Check sheet for the modelled part. Datum: model origin and axes. Units: mm. Coordinates: 2 decimals unless noted, no trailing zeros. Loops run counter-clockwise (first coordinate to the right, second up) from the corner with the lowest first, then second, coordinate; pieces in that order, holes last. Notation, with made-up numbers: (-0.5, 42.5) -> (28.5, 42.5) arc R10 ccw to (28.5, 59.5) -> close; hole circle Ø10 at (21, 28.5). An arc over 180 degrees is marked (long way). Use one line per item in the form item = value.
Autodesk Inventor part; units mm, degrees
ref_plane "YZ Plane" through (0, 0, 0) normal (1, 0, 0) x (0, 1, 0)
ref_plane "XZ Plane" through (0, 0, 0) normal (0, 1, 0) x (-1, 0, 0)
ref_plane "XY Plane" through (0, 0, 0) normal (0, 0, 1) x (1, 0, 0)
sketch "スケッチ1" plane through (0, 0, 0) normal (0, 1, 0) x (-1, 0, 0)
  circle A0 centre (0, 0) radius 5.05
  line L0 (-8.5, 0) -> (8.5, 0) construction
  circle A1 centre (-8.5, 0) radius 1.35
  circle A2 centre (-6.0104, -6.0104) radius 1.35
  circle A3 centre (0, -8.5) radius 1.35
  circle A4 centre (6.0104, -6.0104) radius 1.35
  circle A5 centre (0, -145.8097) radius 16 construction
  line L1 (0, 0) -> (0, -145.8097) construction
  arc A6 (-20.3699, -115.9088) -> (20.3699, -115.9088) centre (0, -145.8097) ccw
  circle A7 centre (-8.5, 0) radius 2.4 construction
  line L2 (-16, 31) -> (16, 31) construction
  line L3 (16, 31) -> (16, -12) construction
  line L4 (16, -12) -> (-16, -12) construction
  line L5 (-16, -12) -> (-16, 31) construction
  line L6 (-16, 31) -> (16, -12) construction
  line L7 (16, 31) -> (-16, -12) construction
  arc A8 (-16, 0) -> (-10.583, -12) centre (0, 0) ccw construction
  arc A9 (10.583, -12) -> (16, 0) centre (0, 0) ccw construction
  line L8 (-16, -107.6443) -> (-16, 0)
  line L9 (16, -107.6443) -> (16, 0)
  circle A10 centre (0, -82.5) radius 1.6
  line L10 (0, -145.8097) -> (-25.5832, -120.2265) construction
  circle A11 centre (-22.7548, -123.055) radius 4 construction
  circle A12 centre (-22.7548, -123.055) radius 1.6
  circle A13 centre (-22.7548, -168.5645) radius 1.6
  circle A14 centre (22.7548, -168.5645) radius 1.6
  circle A15 centre (22.7548, -123.055) radius 1.6
  line L11 (30.6064, -21.0119) -> (2.8936, -37.0119) construction
  line L12 (2.8936, -37.0119) -> (-18.6064, 0.2272) construction
  line L13 (-18.6064, 0.2272) -> (9.1064, 16.2272) construction
  line L14 (9.1064, 16.2272) -> (30.6064, -21.0119) construction
  line L15 (30.6064, -21.0119) -> (-18.6064, 0.2272) construction
  line L16 (2.8936, -37.0119) -> (9.1064, 16.2272) construction
  line L17 (16.75, -29.0119) -> (-4.75, 8.2272) construction
  circle A16 centre (0, -42.5) radius 1.6
  line L18 (-2.5, -47.5) -> (2.5, -47.5) construction
  line L19 (2.5, -47.5) -> (2.5, -57.5) construction
  line L20 (2.5, -57.5) -> (-2.5, -57.5) construction
  line L21 (-2.5, -57.5) -> (-2.5, -47.5) construction
  line L22 (-2.5, -47.5) -> (2.5, -57.5) construction
  line L23 (2.5, -47.5) -> (-2.5, -57.5) construction
  line L24 (-2.5, -52.5) -> (2.5, -52.5) construction
  circle A17 centre (0, -62.5) radius 1.6
  line L25 (2.8936, -37.0119) -> (49.2811, -117.3573) construction
  line L26 (0, -145.8097) -> (49.2811, -117.3573) construction
  line L27 (-2.5, -47.5) -> (2.5, -47.5) construction
  line L28 (2.5, -47.5) -> (2.5, -77.5) construction
  line L29 (2.5, -77.5) -> (-2.5, -77.5) construction
  line L30 (-2.5, -77.5) -> (-2.5, -47.5) construction
  line L31 (-2.5, -47.5) -> (2.5, -77.5) construction
  line L32 (2.5, -47.5) -> (-2.5, -77.5) construction
  line L33 (-2.55, -47.45) -> (2.55, -47.45)
  line L34 (2.55, -47.45) -> (2.55, -77.55)
  line L35 (2.55, -77.55) -> (-2.55, -77.55)
  line L36 (-2.55, -77.55) -> (-2.55, -47.45)
  line L37 (-2.55, -47.45) -> (2.55, -77.55) construction
  line L38 (2.55, -47.45) -> (-2.55, -77.55) construction
  arc A18 (-1.0651, -47.45) -> (-2.55, -48.9349) centre (-1.8075, -48.1925) ccw
  arc A19 (2.55, -48.9349) -> (1.0651, -47.45) centre (1.8075, -48.1925) ccw
  line L39 (-2.5, -62.5) -> (2.5, -62.5) construction
  arc A20 (-2.55, -76.0651) -> (-1.0651, -77.55) centre (-1.8075, -76.8075) ccw
  arc A21 (1.0651, -77.55) -> (2.55, -76.0651) centre (1.8075, -76.8075) ccw
  arc A22 (16, 0) -> (8.0571, 13.8233) centre (0, 0) ccw
  circle A23 centre (0, -145.8097) radius 28.1801
  line L40 (-5.05, 0) -> (-5.05, 12.0954)
  line L41 (5.05, 0) -> (5.05, 12.0954)
  circle A24 centre (8.5, 0) radius 1.35
  arc A25 (-8.0571, 13.8233) -> (-16, 0) centre (0, 0) ccw
  arc A26 (-5.05, 12.0954) -> (-8.0571, 13.8233) centre (-7.05, 12.0954) ccw
  arc A27 (8.0571, 13.8233) -> (5.05, 12.0954) centre (7.05, 12.0954) ccw
  arc A28 (-20.3699, -115.9088) -> (-16, -107.6443) centre (-26, -107.6443) ccw
  arc A29 (16, -107.6443) -> (20.3699, -115.9088) centre (26, -107.6443) ccw
  point P0 (0, 9.5)
  point P1 (0, 9.5)
  point P2 (-16, -113.3598)
  point P3 (16, -113.3598)
  point P4 (6, -10.3923)
  point P5 (0, -52.5)
  point P6 (0, -62.5)
  point P7 (1.0651, -77.55)
  point P8 (-1.0651, -77.55)
  point P9 (-2.55, -76.0651)
  point P10 (2.55, -48.9349)
  point P11 (2.55, -76.0651)
  point P12 (0, -181.9899)
  point P13 (-5.05, 15.1821)
  point P14 (5.05, 15.1821)
  point P15 (5.05, 9.6596)
  point P16 (5.05, 0)
  dimension "d0" = 10.1
  dimension "d1" = 17
  dimension "d2" = 2.7
  dimension "d5" = 180
  dimension "d7" = 32
  dimension "d8" = 145.8098
  dimension "d9" = 72.3602
  dimension "d10" = 4.8
  dimension "d11" = 32
  dimension "d12" = 43
  dimension "d14" = 9.5
  dimension "d17" = 3.2
  dimension "d23" = 32
  dimension "d24" = 45
  dimension "d25" = 8
  dimension "d26" = 3.2
  dimension "d29" = 360
  dimension "d33" = 32
  dimension "d34" = 43
  dimension "d36" = 9.5
  dimension "d37" = 150
  dimension "d38" = 3.2
  dimension "d40" = 5
  dimension "d41" = 10
  dimension "d42" = 40
  dimension "d43" = 20
  dimension "d44" = 42.5
  dimension "d45" = 30
  dimension "d46" = 1.05
  dimension "d47" = 0.05
  dimension "d48" = 0.05
  dimension "d49" = 16
  dimension "d50" = 181.9898
  dimension "d53" = 90
  dimension "d54" = 2
  dimension "d55" = 10
extrude "押し出し1" add sketch "スケッチ1" along normal blind 2 contours L41 A27 A22 L9 A29 A6 A28 L8 A25 A26 L40 A0
properties part number "ForeArm_outside_frame" material "GFRP"
(1) Go/stop test with flat-tipped pins: P1, Ø0.6, axis at y = 1, z = -31, coming from the +X side; P2, Ø1, axis at y = 0.5, z = 3.5, coming from the -X side; P3, Ø2, axis at x = 6.01, z = -6.01, coming from the -Y side; P4, Ø0.6, axis at y = 1.5, z = -54.5, coming from the -X side. Record where each tip stops, or that it passes through.
Established:
P1 = 16
P2 = -15.72
P3 = through
P4 = -16
(2) Section check D-D, the plane z = -104.5. Record the boundary of the cut face in (x, y), plus the area to 3 significant figures.
Established:
outline = (-16, 0) -> (16, 0) -> (16, 2) -> (-16, 2) -> close
area = 64.0 mm²
(3) Section check C-C, the plane x = -13. Record the boundary of the cut face in (y, z), plus the area to 3 significant figures.
Established:
outline = (0, -179.57) -> (2, -179.57) -> (2, -170.81) -> (0, -170.81) -> close; (0, -120.81) -> (2, -120.81) -> (2, 9.33) -> (0, 9.33) -> close
area = 278 mm²
(4) Scan lines: line 1 along Z through (x, y) = (0, 0.85); line 2 along Z through (x, y) = (2, 0.2); line 3 along Z through (x, y) = (-2.5, 0.3). Record each from-to range of solid material in increasing order.
Established:
line_1 = -181.99 to -173.99, -117.63 to -84.1, -80.9 to -77.55, -47.45 to -44.1, -40.9 to -9.85, -7.15 to -5.05
line_2 = -181.93 to -173.92, -117.7 to -77.84, -47.16 to -4.64
line_3 = -181.9 to -173.88, -117.74 to -77.6, -47.4 to -4.39
(5) Section check A-A, the plane z = -69. Record the boundary of the cut face in (x, y), plus the area to 3 significant figures.
Established:
outline = (-16, 0) -> (-2.55, 0) -> (-2.55, 2) -> (-16, 2) -> close; (2.55, 0) -> (16, 0) -> (16, 2) -> (2.55, 2) -> close
area = 53.8 mm²
(6) Section check B-B, the plane y = 1.7. Give the number of separate pieces and of enclosed holes in the cut face, plus the area to 3 significant figures.
Established:
separate_pieces = 1
enclosed_holes = 13
area = 5,140 mm²
